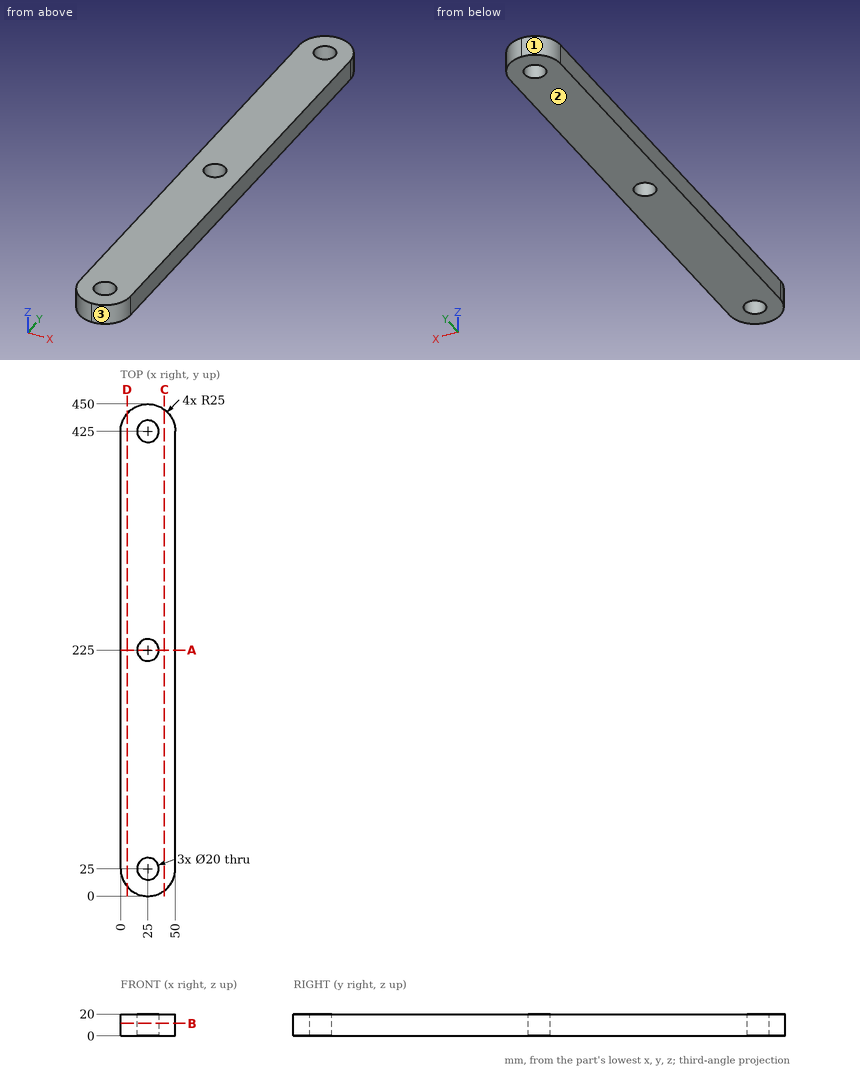
Design review of the part shown in the three views and the two pictorial views. Dimensions are in mm from the part's minimum x, y and z. Round coordinates to 2 decimals unless told otherwise and drop trailing zeros. Write each loop counter-clockwise with the first axis right and the second up, starting at its lowest first coordinate (ties: lowest second). Pieces come first, ordered by that corner, then holes. Notation, with made-up numbers: (-32, -34) -> (20, -34) arc R12 ccw to (20, -13) -> close; hole circle Ø5 at (45.25, 56.25). An arc over 180 degrees is marked (long way). Answer as a JSON object with one key per item and string values.
1. To check wall thickness, follow line 1 along Y through (x, z) = (25, 15.75); line 2 along X through (y, z) = (425, 8.75); line 3 along X through (y, z) = (430.5, 2.75). State the ranges of each line that lie inside material, in increasing order.
Results found:
{"line 1": "y = 0 to 15, 35 to 215, 235 to 415, 435 to 450", "line 2": "x = 0 to 15, 35 to 50", "line 3": "x = 0.61 to 16.65, 33.35 to 49.39"}
2. We need section A-A on y = 225. State the section outline as (x, z) points.
Results found:
{"outline": "(0, 0) -> (15, 0) -> (15, 20) -> (0, 20) -> close; (35, 0) -> (50, 0) -> (50, 20) -> (35, 20) -> close"}
3. We need section C-C on x = 40. State the section outline as (y, z) points, and give its area (3 significant figures).
Results found:
{"outline": "(5, 0) -> (445, 0) -> (445, 20) -> (5, 20) -> close", "area": "8,800 mm^2"}
4. We need section D-D on x = 6. State the section outline as (y, z) points.
Results found:
{"outline": "(8.75, 0) -> (441.25, 0) -> (441.25, 20) -> (8.75, 20) -> close"}
5. Clearance check with flat-ended pins moving along their axes: pin 1 (10 mm diameter, centred on x = 34.5, z = 7, fed in from -Y); pin 2 (18 mm diameter, centred on x = 25, y = 225, fed in from +Z); pin 3 (4 mm diameter, centred on x = 34, z = 4.5, fed in from -Y); pin 4 (4 mm diameter, centred on x = 18.5, z = 15, fed in from +Y). State where each tip first meets the part, or that it passes through.
Results found:
{"pin 1": "stops at y = 0.41", "pin 2": "passes through", "pin 3": "stops at y = 1", "pin 4": "stops at y = 449.59"}
6. We need section B-B on z = 11.5. State how many separate pieces and enclosed holes the cut face has, and give its area (3 significant figures).
Results found:
{"separate pieces": "1", "enclosed holes": "3", "area": "21,000 mm^2"}
7. The part is to be moulded in two halves that separate along Y. For the marked faces 1, 2 and 3, say which applies: pulls with the +Y half, pulls with the -Y half, needs draft (parallel to the pull), parting line crosses it, or undercut.
Results found:
{"face 1": "pulls with the +Y half", "face 2": "needs draft", "face 3": "pulls with the -Y half"}
